Could you check a few things on this model? Use its own coordinates, in mm. Give positions to 0.01 mm unless a question says otherwise; leave off trailing zeros. Order: outer loops, then holes, each group sorted by start corner. A loop starts at its lowest first (then second) coordinate and runs counter-clockwise, first axis right, second up. Notation, with made-up numbers: (56.25, -38.5) -> (62.25, -38.5) arc R32 cw to (62.25, 0.5) -> close; hole circle Ø11 at (16, 57.5). An arc over 180 degrees is marked (long way). Answer as CSV lines item,"result". Start each with the question number.
(1) I need wall thicknesses on L1, parallel to X at y = -4.25, z = -118.5; L2, parallel to X at y = -12.75, z = -91.5; L3, parallel to Z at x = -573, y = -8.5. Which ranges of each line are inside material? Lowest first, please.
(2) I want a section at C-C (z = 158). Please give me the cut outline in (x, y), plus the area to 3 significant figures.
(3) I want a section at B-B (z = -211.5). Please give me the cut outline in (x, y).
(4) I want a section at A-A (y = -5.75). Please give me the cut outline in (x, z), plus the area to 3 significant figures.
(5) Will these pins go through, and if not, where does the flat tip stop? pin 1 Ø10 at (y, z) = (-9, -138.5) entering from -X; pin 2 Ø1.5 at (y, z) = (-12.5, -116.5) entering from -X.
(6) We'd pull the mould along X, two halves only. Please class faces 1 (the face through (-303, 0, -76)), 2 (the face through (-653.19, -9.66, -79.78)), 3 (the face through (-803.32, -9.39, -263.36)): released by +X, released by -X, zero draft, split by the parting line, or undercut.
```python
from build123d import *

# Parameters (mm, degrees)
F1_DEPTH = 19.05
F2_R     = 45.72
F3_DEPTH = 25.4


with BuildPart() as f1:
    # F0 (on Front) → F1 (new body)
    with BuildSketch(Plane.XZ):
        Polygon((-690.083177, 286.513845), (-913.432107, -81.786155), (-690.083177, -450.086155), (-563.697045, -449.713886), (198.302955, -449.713886), (325.572278, -449.713886), (325.572278, 286.886114), (198.572278, 286.886114), (198.302955, 286.886114), (-563.697045, 286.886114), align=None)
        Polygon((-563.697045, -449.713886), (-690.083177, -450.086155), (325.572278, -450.086155), (325.572278, -449.713886), (198.302955, -449.713886), align=None)
        Polygon((-690.083177, 286.886114), (-690.083177, 286.513845), (-563.697045, 286.886114), align=None)
    extrude(amount=F1_DEPTH)

    # F2 (on face) → F3 (cut)
    with BuildSketch(Plane.XZ.offset(19.05)):
        with Locations((-607.512472, -81.786155)):
            Circle(F2_R)
    extrude(amount=-F3_DEPTH, mode=Mode.SUBTRACT)


solid = f1.part
```
Final values:
1,L1,"-891.17 to -634.76, -580.27 to 325.57"
1,L2,"-907.54 to -652.19, -562.84 to 325.57"
1,L3,"-450.09 to -111.77, -51.8 to 286.89"
2,outline,"(-768.02, -19.05) -> (325.57, -19.05) -> (325.57, 0) -> (-768.02, 0) -> close"
2,area,"20,800 mm²"
3,outline,"(-834.77, -19.05) -> (325.57, -19.05) -> (325.57, 0) -> (-834.77, 0) -> close"
4,outline,"(-913.43, -81.79) -> (-690.08, -450.09) -> (325.57, -450.09) -> (325.57, 286.89) -> (-690.08, 286.89) -> (-690.08, 286.51) -> close; hole circle Ø91.44 at (-607.51, -81.79)"
4,area,"824,000 mm²"
5,pin 1,"x = -882.07"
5,pin 2,"x = -892.84"
6,face 1,"zero draft"
6,face 2,"undercut"
6,face 3,"released by -X"
